Input: dimensioned drawing with shaded views. Units: mm. Origin: part minimum x, y, z. A direction names the side the tool comes from. Coordinates: 2 decimals unless noted, no trailing zeros. Order: outer loops, then holes, each group sorted by start corner. A loop starts at its lowest first (then second) coordinate and runs counter-clockwise, first axis right, second up. Notation, with made-up numbers: (13, -33) -> (64, -33) arc R12 ccw to (64, -20) -> close; hole circle Ø7 at (79, 1.5). An arc over 180 degrees is marked (long way). Write item = value, one per line. Start each with the question number.
Item 1: Section query B-B (z = 137). Output: boundary loops of the cut face in (x, y), then the cut area to 3 significant figures.
Item 2: Ray query, line 1 along Y through (x, z) = (224, 98.5); line 2 along Y through (x, z) = (151, 23); line 3 along X through (y, z) = (30.5, 41). Return the intervals inside material, ascending. Write a range as [from, to].
Item 3: Section query D-D (z = 26). Output: boundary loops of the cut face in (x, y).
Item 4: Set-up query: the marked faces 1 and 2. Return all of +Z, -Z, +X, -X, +Y, -Y with unobstructed straight access to the full face (end or side cutting, diameter ignored); none if empty.
Item 5: Section query C-C (y = 27). Output: boundary loops of the cut face in (x, z).
Item 6: Section query A-A (x = 137). Output: boundary loops of the cut face in (y, z), then the cut area to 3 significant figures.
Item 7: Contact query for flat-ended pins moving along their axis: pin 1 (1.5 mm diameter, centred on y = 11, z = 195, fed in from +X); pin 2 (3 mm diameter, centred on y = 19, z = 165, fed in from +X); pin 3 (4 mm diameter, centred on x = 180, y = 19.5, fed in from -Z). Output: stop coordinate, or through.
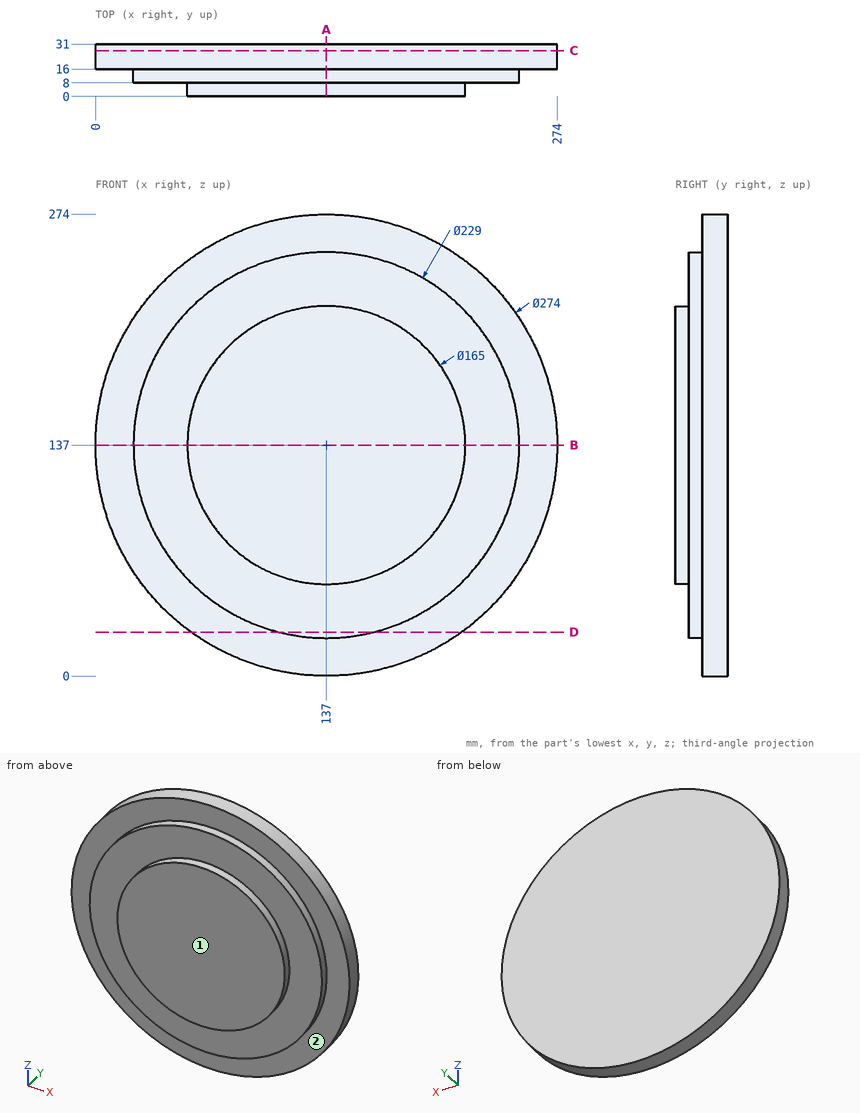
Computed:
q1.outline = (0, 16) -> (22.5, 16) -> (22.5, 8) -> (54.5, 8) -> (54.5, 0) -> (219.5, 0) -> (219.5, 8) -> (251.5, 8) -> (251.5, 16) -> (274, 16) -> (274, 31) -> (0, 31) -> close
q1.area = 7,260 mm^2
q2.line_1 = [8, 31]
q2.line_2 = [16, 31]
q2.line_3 = [39.26, 234.74]
q3.outline = (56.7, 16) -> (108.91, 16) -> (108.91, 8) -> (165.09, 8) -> (165.09, 16) -> (217.3, 16) -> (217.3, 31) -> (56.7, 31) -> close
q4.face_1 = +Z, -Z, +X, -X, -Y
q4.face_2 = -Y
q5.outline = circle Ø274 at (137, 137)
q6.outline = (0, 54.5) -> (8, 54.5) -> (8, 22.5) -> (16, 22.5) -> (16, 0) -> (31, 0) -> (31, 274) -> (16, 274) -> (16, 251.5) -> (8, 251.5) -> (8, 219.5) -> (0, 219.5) -> close
q6.area = 7,260 mm^2
q7.pin_1 = 236.16
q7.pin_2 = 271.41
q7.pin_3 = 6.28
